```python
from build123d import *

# Parameters (mm, degrees)
SKETCH1_W           = 60
SKETCH1_H           = 40
BOSS_EXTRUDE1_DEPTH = 38.1


with BuildPart() as part:
    # Sketch1 → Boss-Extrude1 (new body)
    with BuildSketch(Plane(origin=(0, 0, 0), x_dir=(1, 0, 0), z_dir=(0, 1, 0))):
        Rectangle(SKETCH1_W, SKETCH1_H)
    extrude(amount=-BOSS_EXTRUDE1_DEPTH)

    # Sketch2 → Cut-Revolve1 (revolve, cut)
    with BuildSketch(Plane.XY, mode=Mode.PRIVATE) as cut_revolve1_sk:
        Polygon((62.630929862, -36.1), (62.630929862, -23.4), (5, -23.4), (12.630929862, -36.1), align=None)
        Polygon((-12.630929862, -36.1), (-5, -23.4), (-62.630929862, -23.4), (-62.630929862, -36.1), align=None)
    revolve(cut_revolve1_sk.sketch.rotate(Axis((-5, -23.4, 0), (-1, 0, 0)), 180), axis=Axis((-5, -23.4, 0), (-1, 0, 0)), mode=Mode.SUBTRACT)

    # Sketch4 → Cut-Revolve2 (revolve, cut)
    with BuildSketch(Plane.XY):
        Polygon((-17.5, -11), (-17.5, -38.1), (0, -38.1), (0, -2), (-11, -2), (-11, -3), (-13, -3), (-13, -11), align=None)
    revolve(axis=Axis((0, -2, 0), (0, -1, 0)), mode=Mode.SUBTRACT)


solid = part.part
```
Model file for the job. Use its own axes, mm. A direction names the side the tool comes from. Coordinates: 2 decimals unless noted, no trailing zeros. Loops run counter-clockwise (first coordinate to the right, second up) from the corner with the lowest first, then second, coordinate; pieces in that order, holes last. Notation, with made-up numbers: (56, -22) - (80, -22) arc R33 ccw to (80, 13) - close; hole circle Ø4 at (-12.5, -37.75). An arc over 180 degrees is marked (long way). Write item = value, one per line. Start each with the question number.
Item 1: Saw through at B-B, the plane x = 0. List the corners of the cut face in (y, z), then the cut area to 4 significant figures.
Item 2: Saw through at D-D, the plane x = 21.5. List the corners of the cut face in (y, z).
Item 3: Wall check: probe 1 along Z at (x, y) = (25, -23.4); probe 2 along Z at (x, y) = (0, -3.5); probe 3 along X at (y, z) = (-4, 10). Give the ranges that are in metal, low to high. Write a range as [from, to].
Item 4: Saw through at C-C, the plane y = -31. List the corners of the cut face in (x, z), then the cut area to 3 significant figures.
Item 5: Drop flat-ended pins along their axis: pin 1 Ø21 at (x, z) = (-1, 0.5) entering from -Y; pin 2 Ø17.5 at (x, z) = (1.5, -1.5) entering from -Y; pin 3 Ø12 at (x, z) = (-2.5, -8.5) entering from -Y. Give the stop position or say it passes through.
Item 6: Saw through at A-A, the plane z = 0. List the corners of the cut face in (x, y), then the cut area to 3 significant figures.
Item 7: 3-axis set-ups, long thin cutter, end or side, ignore diameter. For faces 1 (the face through (0, -2, 0)), 2 (the face through (-23.124, -11.668, 4.864)), 3 (the face through (-30, -10, 0)): which of +Z, -Z, +X, -X, +Y, -Y reach the whole face in a straight line?
Item 8: Pull direction Y, two halves, no side cores. Call faces 4 (the face through (2.38, -2.51, 10.74)), 5 (the face through (23.367, -17.54, 11.267)), 6 (the face through (-11, -3, -3)): +Y half, -Y half, draft (parallel to the pull), parting line (faces both ways), or undercut.
Answers:
q1.outline = (-38.1, -20) - (0, -20) - (0, 20) - (-38.1, 20) - (-38.1, 17.5) - (-11, 17.5) - (-11, 13) - (-3, 13) - (-3, 11) - (-2, 11) - (-2, -11) - (-3, -11) - (-3, -13) - (-11, -13) - (-11, -17.5) - (-38.1, -17.5) - close
q1.area = 345.5 mm2
q2.outline = (-38.1, -20) - (0, -20) - (0, 20) - (-38.1, 20) - close; hole circle Ø25.4 at (-23.4, 0)
q3.probe_1 = [-20, -12.7], [12.7, 20]
q3.probe_2 = [-20, -13], [13, 20]
q3.probe_3 = [-30, -8.31], [8.31, 30]
q4.outline = (-30, -20) - (30, -20) - (30, -10.17) - (14.24, -10.17) arc R17.5 cw to (-14.24, -10.17) - (-30, -10.17) - close; (-30, 10.17) - (-14.24, 10.17) arc R17.5 cw to (14.24, 10.17) - (30, 10.17) - (30, 20) - (-30, 20) - close
q4.area = 887 mm2
q5.pin_1 = -3
q5.pin_2 = -2
q5.pin_3 = -11
q6.outline = (-30, -38.1) - (-17.5, -38.1) - (-17.5, -36.1) - (-30, -36.1) - close; (-30, -10.7) - (-13, -10.7) - (-13, -3) - (-11, -3) - (-11, -2) - (11, -2) - (11, -3) - (13, -3) - (13, -10.7) - (30, -10.7) - (30, 0) - (-30, 0) - close; (17.5, -38.1) - (30, -38.1) - (30, -36.1) - (17.5, -36.1) - close
q6.area = 470 mm2
q7.face_1 = -Y
q7.face_2 = -X
q7.face_3 = +Z, -Z, -X, +Y, -Y
q8.face_4 = draft
q8.face_5 = undercut
q8.face_6 = -Y half
